```python
from build123d import *

# Parameters (mm, degrees)
BOSS_EXTRUDE1_DEPTH             = 10
BOSS_EXTRUDE2_DEPTH             = 9
CBORE_FOR_M5_SBHCS1_D           = 5.5
CBORE_FOR_M5_SBHCS1_CBORE_D     = 10.5
CBORE_FOR_M5_SBHCS1_CBORE_DEPTH = 2.75
CBORE_FOR_M5_SBHCS2_D           = 5.5
CBORE_FOR_M5_SBHCS2_CBORE_D     = 10.5
CBORE_FOR_M5_SBHCS2_CBORE_DEPTH = 2.75
CBORE_FOR_M3_SBHCS1_D           = 3.4
CBORE_FOR_M3_SBHCS1_CBORE_D     = 6.7
CBORE_FOR_M3_SBHCS1_CBORE_DEPTH = 16
CBORE_FOR_M3_SBHCS2_D           = 3.4
CBORE_FOR_M3_SBHCS2_CBORE_D     = 6.7
CBORE_FOR_M3_SBHCS2_CBORE_DEPTH = 6
F_5_4_5_4_DIAMETER_HOLE1_D      = 5.4


with BuildPart() as part:
    # Sketch1 → Boss-Extrude1 (new body)
    with BuildSketch(Plane(origin=(0, 0, 0), x_dir=(1, 0, 0), z_dir=(0, 1, 0))):
        Polygon((0, 0), (60, 0), (60, 40), (20, 40), (20, 20), (0, 20), align=None)
    extrude(amount=BOSS_EXTRUDE1_DEPTH)

    # Sketch2 → Boss-Extrude2 (add)
    with BuildSketch(Plane(origin=(0, 10, 0), x_dir=(1, 0, 0), z_dir=(0, 1, 0))):
        Polygon((20, 40), (7, 40), (7, 20), (0, 20), (0, 0), (60, 0), (60, 40), align=None)
    extrude(amount=BOSS_EXTRUDE2_DEPTH)

    # CBORE for M5 SBHCS1 (through all)
    with Locations(Plane(origin=(0, 19, 0), x_dir=(1, 0, 0), z_dir=(0, 1, 0))):
        with Locations((10, 7.5), (30, 7.5), (30, 32.5)):
            CounterBoreHole(CBORE_FOR_M5_SBHCS1_D / 2, CBORE_FOR_M5_SBHCS1_CBORE_D / 2, CBORE_FOR_M5_SBHCS1_CBORE_DEPTH)

    # CBORE for M5 SBHCS2 (through all)
    with Locations(Plane(origin=(0, 19, 0), x_dir=(1, 0, 0), z_dir=(0, 1, 0))):
        with Locations((52.5, 30), (52.5, 10)):
            CounterBoreHole(CBORE_FOR_M5_SBHCS2_D / 2, CBORE_FOR_M5_SBHCS2_CBORE_D / 2, CBORE_FOR_M5_SBHCS2_CBORE_DEPTH)

    # CBORE for M3 SBHCS1 (through all)
    with Locations(Plane(origin=(0, 0, 0), x_dir=(-1, 0, 0), z_dir=(0, -1, 0))):
        with Locations((-30, 20)):
            CounterBoreHole(CBORE_FOR_M3_SBHCS1_D / 2, CBORE_FOR_M3_SBHCS1_CBORE_D / 2, CBORE_FOR_M3_SBHCS1_CBORE_DEPTH)

    # CBORE for M3 SBHCS2 (through all)
    with Locations(Plane(origin=(0, 10, 0), x_dir=(-1, 0, 0), z_dir=(0, -1, 0))):
        with Locations((-13.5, 33)):
            CounterBoreHole(CBORE_FOR_M3_SBHCS2_D / 2, CBORE_FOR_M3_SBHCS2_CBORE_D / 2, CBORE_FOR_M3_SBHCS2_CBORE_DEPTH)

    # Ø5.4 (5.4) Diameter Hole1 (through all)
    with Locations(Plane(origin=(0, 0, 0), x_dir=(-1, 0, 0), z_dir=(0, -1, 0))):
        with Locations((-13.5, 20)):
            Hole(F_5_4_5_4_DIAMETER_HOLE1_D / 2)


with BuildPart() as body_2:
    # Mirror1: mirrored copy
    add(part.part.mirror(Plane(origin=(60, 10, 0), x_dir=(0, 0, 1), z_dir=(-1, 0, 0))))


solid = body_2.part
```
The model under review builds one solid part; all positions refer to its coordinate system, in mm. A direction names the side the tool comes from. Give positions to 0.01 mm unless a question says otherwise; leave off trailing zeros. Write each loop counter-clockwise with the first axis right and the second up, starting at its lowest first coordinate (ties: lowest second). Pieces come first, ordered by that corner, then holes. Notation, with made-up numbers: M 30,47 L 71,47 A24 cw 71,77 Z; hole C 70,31 d6. An arc over 180 degrees is marked long. Answer in a Markdown table with one row per item.
Item 1: Tool access review of faces 5 (the face through (60, 9, -20)), 6 (the face through (71.37, 17.64, -33.55)), 7 (the face through (107.85, 17.52, -31.97)), 8 (the face through (106, 16, -35)), 9 (the face through (100, 5, -30)): name each direction out of +Z, -Z, +X, -X, +Y, -Y from which nothing blocks a thin tool from reaching the whole face with its end or side.
Check sheet entries:
| item | result |
|---|---|
| face 5 | +Z, -Z, -X, +Y, -Y |
| face 6 | +Y |
| face 7 | +Y, -Y |
| face 8 | -Y |
| face 9 | -Z, +X, -Y |
Item 2: Add section B-B on y = 13.75. State how many separate pieces and enclosed holes the cut face has, plus the area to 3 significant figures.
Check sheet entries:
| item | result |
|---|---|
| separate pieces | 1 |
| enclosed holes | 8 |
| area | 2,050 mm2 |
Item 3: Add section A-A on x = 67.5. Give the boundary of the cut face in (y, z), plus the area to 4 significant figures.
Check sheet entries:
| item | result |
|---|---|
| outline | M 0,-40 L 19,-40 L 19,-35.25 L 16.25,-35.25 L 16.25,-32.75 L 0,-32.75 Z; M 0,-27.25 L 16.25,-27.25 L 16.25,-24.75 L 19,-24.75 L 19,-15.25 L 16.25,-15.25 L 16.25,-12.75 L 0,-12.75 Z; M 0,-7.25 L 16.25,-7.25 L 16.25,-4.75 L 19,-4.75 L 19,0 L 0,0 Z |
| area | 523.5 mm2 |
Item 4: Draft analysis for pull direction X (two halves, no side actions). For faces 1 (the face through (113, 14, -30)), 2 (the face through (116, 9, -20)), 3 (the face through (87.253, 8.011, -7.621)), 4 (the face through (88, 16.25, -30)), state which applies: +X half, -X half, draft (parallel to the pull), parting line (faces both ways), or undercut.
Check sheet entries:
| item | result |
|---|---|
| face 1 | +X half |
| face 2 | draft |
| face 3 | undercut |
| face 4 | undercut |
Item 5: Add section C-C on z = -28.5. Give the boundary of the cut face in (x, y).
Check sheet entries:
| item | result |
|---|---|
| outline | M 60,0 L 65.2,0 L 65.2,16.25 L 62.47,16.25 L 62.47,19 L 60,19 Z; M 69.8,0 L 100,0 L 100,10 L 113,10 L 113,19 L 93.4,19 L 93.4,16.25 L 86.6,16.25 L 86.6,19 L 72.53,19 L 72.53,16.25 L 69.8,16.25 Z |
Item 6: Add section D-D on y = 2.5. Give the boundary of the cut face in (x, z), plus the area to 3 significant figures.
Check sheet entries:
| item | result |
|---|---|
| outline | M 60,-40 L 100,-40 L 100,-20 L 103.8,-20 A2.7 cw 109.2,-20 L 120,-20 L 120,0 L 60,0 Z; hole C 67.5,-30 d5.5; hole C 67.5,-10 d5.5; hole C 90,-20 d6.7; hole C 90,-32.5 d5.5; hole C 90,-7.5 d5.5; hole C 110,-7.5 d5.5 |
| area | 1,830 mm2 |
Item 7: For line 1 along Z through (x, y) = (90, 18.1); line 2 along Z through (x, y) = (104.5, 11.25); line 3 along X through (y, z) = (12.75, -32.5), list the stretches that pass through material, from the lowest coordinate up.
Check sheet entries:
| item | result |
|---|---|
| line 1 | -40 to -37.75, -27.25 to -21.7, -18.3 to -12.75, -2.25 to 0 |
| line 2 | -40 to -35.69, -30.31 to -21.81, -18.19 to 0 |
| line 3 | 60 to 66.35, 68.65 to 87.25, 92.75 to 103.19, 109.81 to 113 |
Item 8: For P1, Ø9, axis at x = 90, z = -7.5, coming from the +Y side; P2, Ø5.5, axis at x = 112, y = 9.5, coming from the -Z side; P3, Ø1, axis at y = 6, z = -27, coming from the +X side; P4, Ø5.5, axis at x = 106, z = -33.5, coming from the -Y side, all flat-tipped, find the tip position at first contact; note any pin that passes through.
Check sheet entries:
| item | result |
|---|---|
| P1 | y = 16.25 |
| P2 | z = -40 |
| P3 | x = 100 |
| P4 | y = 10 |
